```python
from build123d import *

# Parameters (mm, degrees)
SKETCH_1_R          = 20
SKETCH_1_R_2        = 1.6
SKETCH_1_R_3        = 1.55
SKETCH_1_R_4        = 2
EXTRUDE_1_DEPTH     = 3
SKETCH_2_R          = 11.5
SKETCH_2_R_2        = 10.5
EXTRUDE_2_DEPTH     = 3
SKETCH_3_R          = 1.9
CUT_EXTRUDE_1_DEPTH = 3


with BuildPart() as part:
    # 草图1 → 凸台-拉伸1 (new body)
    with BuildSketch(Plane(origin=(0, 0, 0), x_dir=(1, 0, 0), z_dir=(0, 1, 0))):
        with Locations(Location((0, 0, 0), (0, 0, 270))):
            Circle(SKETCH_1_R)
        with Locations(Location((0, 15, 0), (0, 0, 270))):
            Circle(SKETCH_1_R_2, mode=Mode.SUBTRACT)
        with Locations(Location((15, 0, 0), (0, 0, 270))):
            Circle(SKETCH_1_R_2, mode=Mode.SUBTRACT)
        with Locations(Location((0, -15, 0), (0, 0, 270))):
            Circle(SKETCH_1_R_2, mode=Mode.SUBTRACT)
        with Locations(Location((-15, 0, 0), (0, 0, 270))):
            Circle(SKETCH_1_R_2, mode=Mode.SUBTRACT)
        with Locations(Location((-5, 5, 0), (0, 0, 270))):
            Circle(SKETCH_1_R_3, mode=Mode.SUBTRACT)
        with Locations(Location((5, 5, 0), (0, 0, 270))):
            Circle(SKETCH_1_R_3, mode=Mode.SUBTRACT)
        with Locations(Location((5, -5, 0), (0, 0, 270))):
            Circle(SKETCH_1_R_3, mode=Mode.SUBTRACT)
        with Locations(Location((-5, -5, 0), (0, 0, 270))):
            Circle(SKETCH_1_R_3, mode=Mode.SUBTRACT)
        with Locations(Location((0, 0, 0), (0, 0, 270))):
            Circle(SKETCH_1_R_4, mode=Mode.SUBTRACT)
    extrude(amount=EXTRUDE_1_DEPTH)

    # 草图2 → 凸台-拉伸2 (add)
    with BuildSketch(Plane(origin=(0, 3, 0), x_dir=(1, 0, 0), z_dir=(0, 1, 0))):
        with Locations(Location((0, 0, 0), (0, 0, 270))):
            Circle(SKETCH_2_R)
        with Locations(Location((0, 0, 0), (0, 0, 270))):
            Circle(SKETCH_2_R_2, mode=Mode.SUBTRACT)
    extrude(amount=EXTRUDE_2_DEPTH)

    # 草图3 → 切除-拉伸1 (cut)
    with BuildSketch(Plane.XZ):
        with Locations(Location((0, 15, 0), (0, 0, 270))):
            Circle(SKETCH_3_R)
        with Locations(Location((15, 0, 0), (0, 0, 270))):
            Circle(SKETCH_3_R)
        with Locations(Location((0, -15, 0), (0, 0, 270))):
            Circle(SKETCH_3_R)
        with Locations(Location((-15, 0, 0), (0, 0, 270))):
            Circle(SKETCH_3_R)
    extrude(amount=-CUT_EXTRUDE_1_DEPTH, mode=Mode.SUBTRACT)


solid = part.part
```
Geometry check sheet. Reference: the model listing, model coordinates, mm. A direction names the side the tool comes from. Give positions to 0.01 mm unless a question says otherwise; leave off trailing zeros. Order: outer loops, then holes, each group sorted by start corner. A loop starts at its lowest first (then second) coordinate and runs counter-clockwise, first axis right, second up.
1. Section check D-D, the plane x = 5. Enter the section's corners in (y, z), and give its area (3 significant figures).
2. Section check C-C, the plane z = -15. Enter the section's corners in (x, y), and give its area (3 significant figures).
3. Thickness scan on L1, parallel to X at y = 1.2, z = 0; L2, parallel to Y at x = -16, z = 11.5; L3, parallel to X at y = 4.1, z = 0. Record the ranges inside material, lowest first.
4. Section check B-B, the plane x = 0. Enter the section's corners in (y, z), and give its area (3 significant figures).
5. Release check for a two-part mould opening along X. For faces 3 (the face through (0.08, 1.48, 16.9)), 4 (the face through (-2, 1, 0)), 5 (the face through (-19.524, 1.479, -4.336)), 6 (the face through (-10.2, 6, 3.4)) record: pulls with the +X half, pulls with the -X half, needs draft (parallel to the pull), parting line crosses it, or undercut.
6. Access from +Z, -Z, +X, -X, +Y, -Y to the whole of each face (thin tool, end or side, straight path). Record for faces 1 (the face through (-4.93, 1.48, -6.55)), 2 (the face through (9.7, 4.48, 6.18)).
7. Section check A-A, the plane y = 1.1. Give the number of separate pieces and of enclosed holes in the cut face, and give its area (3 significant figures).
8. Gauge pin test, flat ends, axial feed: pin 1 Ø3 at (x, y) = (-2, 2.5) entering from -Z; pin 2 Ø5 at (x, z) = (15, 0) entering from +Y; pin 3 Ø3 at (y, z) = (3, -14) entering from +X. Record the tip position at first contact, or that the pin passes through.
Values follow:
1. outline: (0, -19.36) - (3, -19.36) - (3, -10.36) - (6, -10.36) - (6, -9.23) - (3, -9.23) - (3, -6.55) - (0, -6.55) - close; (0, -3.45) - (3, -3.45) - (3, 3.45) - (0, 3.45) - close; (0, 6.55) - (3, 6.55) - (3, 9.23) - (6, 9.23) - (6, 10.36) - (3, 10.36) - (3, 19.36) - (0, 19.36) - close
1. area: 104 mm2
2. outline: (-13.23, 0) - (-1.9, 0) - (-1.9, 3) - (-13.23, 3) - close; (1.9, 0) - (13.23, 0) - (13.23, 3) - (1.9, 3) - close
2. area: 68.0 mm2
3. L1: x = -20 to -16.9, -13.1 to -2, 2 to 13.1, 16.9 to 20
3. L2: y = 0 to 3
3. L3: x = -11.5 to -10.5, 10.5 to 11.5
4. outline: (0, -20) - (3, -20) - (3, -16.9) - (0, -16.9) - close; (0, -13.1) - (3, -13.1) - (3, -11.5) - (6, -11.5) - (6, -10.5) - (3, -10.5) - (3, -2) - (0, -2) - close; (0, 2) - (3, 2) - (3, 10.5) - (6, 10.5) - (6, 11.5) - (3, 11.5) - (3, 13.1) - (0, 13.1) - close; (0, 16.9) - (3, 16.9) - (3, 20) - (0, 20) - close
4. area: 91.2 mm2
5. face 3: undercut
5. face 4: undercut
5. face 5: parting line crosses it
5. face 6: needs draft
6. face 1: +Y, -Y
6. face 2: +Y
7. separate pieces: 1
7. enclosed holes: 9
7. area: 1,170 mm2
8. pin 1: stops at z = -19.99
8. pin 2: stops at y = 3
8. pin 3: stops at x = 15.61
